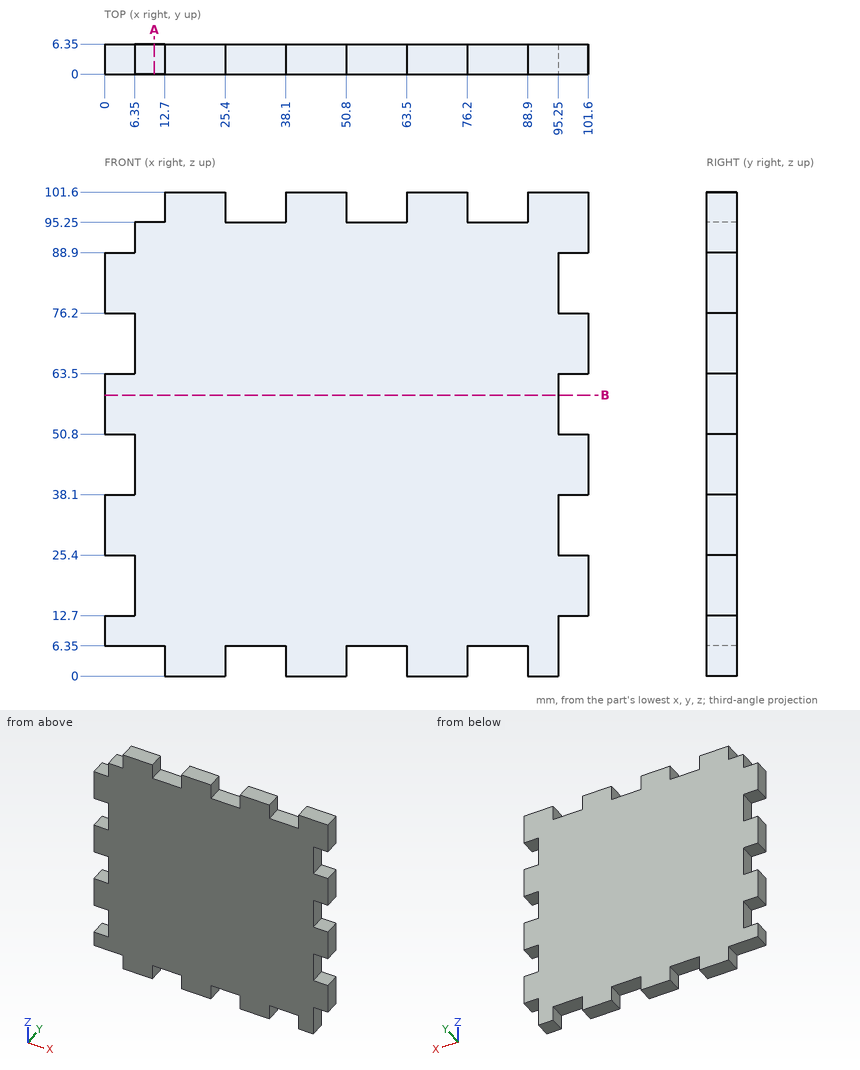
Input: dimensioned drawing with shaded views. Units: mm. Origin: part minimum x, y, z. Give positions to 0.01 mm unless a question says otherwise; leave off trailing zeros. Loops run counter-clockwise (first coordinate to the right, second up) from the corner with the lowest first, then second, coordinate; pieces in that order, holes last. Notation, with made-up numbers: (-2, 52) -> (27, 52) arc R24 ccw to (27, 88) -> close; hole circle Ø2 at (-20.75, 50). An arc over 180 degrees is marked (long way). Use a Markdown table: item, result.
Q1. Section query A-A, the plane x = 10.5. Return the cut outline in (y, z), plus the area to 3 significant figures.
Entries:
| item | result |
|---|---|
| outline | (0, 6.35) -> (6.35, 6.35) -> (6.35, 95.25) -> (0, 95.25) -> close |
| area | 565 mm² |
Q2. Ray query, probe 1 along Z at (x, y) = (5.5, 4.25); probe 2 along Z at (x, y) = (97, 0.5); probe 3 along X at (y, z) = (3.5, 21). Return the intervals inside material, ascending. Write a range as from..to.
Entries:
| item | result |
|---|---|
| probe 1 | z = 6.35..12.7, 25.4..38.1, 50.8..63.5, 76.2..88.9 |
| probe 2 | z = 12.7..25.4, 38.1..50.8, 63.5..76.2, 88.9..101.6 |
| probe 3 | x = 6.35..101.6 |
Q3. Section query B-B, the plane z = 59. Return the cut outline in (x, y), plus the area to 3 significant figures.
Entries:
| item | result |
|---|---|
| outline | (0, 0) -> (95.25, 0) -> (95.25, 6.35) -> (0, 6.35) -> close |
| area | 605 mm² |
Q4. First-contact query: P1, Ø3, axis at x = 8, y = 4, coming from the -Z side; P2, Ø3, axis at x = 3, y = 3, coming from the +Z side; P3, Ø1.9, axis at y = 4.5, z = 2.5, coming from the +X side; P4, Ø1, axis at x = 86.5, z = 38, coming from the -Y side. Flat tips, straight axial feed; report the tip coordinate or a pass-through.
Entries:
| item | result |
|---|---|
| P1 | stops at z = 6.35 |
| P2 | stops at z = 88.9 |
| P3 | stops at x = 95.25 |
| P4 | stops at y = 0 |
